For this review, take the finished solid that the model builds, in its own axes (mm). Coordinates: 2 decimals unless noted, no trailing zeros. Write each loop counter-clockwise with the first axis right and the second up, starting at its lowest first coordinate (ties: lowest second). Pieces come first, ordered by that corner, then holes. Notation, with made-up numbers: (72.25, -23.75) - (119.25, -23.75) arc R32 cw to (119.25, 3.25) - close; hole circle Ø10 at (29, 7). An arc over 180 degrees is marked (long way). Write each question's results on one line, items separated by ' | '.
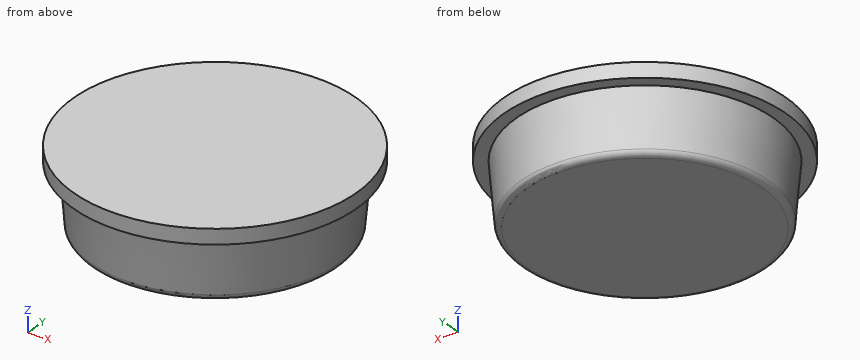
from build123d import *

# Parameters (mm, degrees)
SKETCH2_R           = 6.0325
BOSS_EXTRUDE1_DEPTH = 0.635
SKETCH1_R           = 5.2578
SKETCH3_R           = 5.4864
FILLET1_R           = 0.254


with BuildPart() as part:
    # Sketch2 → Boss-Extrude1 (new body)
    with BuildSketch(Plane.XY.offset(3.302)):
        Circle(SKETCH2_R)
    extrude(amount=-BOSS_EXTRUDE1_DEPTH)

    # Sketch1 → Loft1 section 0
    with BuildSketch(Plane.XY):
        Circle(SKETCH1_R)
    # Sketch3 → Loft1 section 1
    with BuildSketch(Plane(origin=(0, 0, 2.667), x_dir=(-1, 0, 0), z_dir=(0, 0, -1))):
        Circle(SKETCH3_R)
    loft()

    # Fillet1
    fillet1_edges = [part.edges().sort_by_distance(p)[0] for p in [
        (-5.2578, 0, 0),
    ]]
    fillet(fillet1_edges, radius=FILLET1_R)


solid = part.part
Q1. Wall thickness on line 1 along Z through (x, y) = (5.75, 0.5); line 2 along X through (y, z) = (1.75, 1.8); line 3 along X through (y, z) = (3.5, 0.55): over which ranges is each line inside the solid? List them lowest first. Write a range as from..to.
Results found:
line 1: 2.67..3.3 | line 2: -5.12..5.12 | line 3: -3.99..3.99
Q2. Take a section at A-A on x = 0. State the section outline as (y, z) points, plus the area to 3 significant figures.
Results found:
outline: (-6.03, 2.67) - (-5.49, 2.67) - (-5.28, 0.23) arc R0.25 ccw to (-5.02, 0) - (5.02, 0) arc R0.25 ccw to (5.28, 0.23) - (5.49, 2.67) - (6.03, 2.67) - (6.03, 3.3) - (-6.03, 3.3) - close | area: 36.3 mm2
Q3. Take a section at B-B on z = 3. State the section outline as (x, y) points (1 decimal).
Results found:
outline: circle Ø12.1 at (0, 0)
Q4. Take a section at C-C on z = 0.9. State the section outline as (x, y) points.
Results found:
outline: circle Ø10.67 at (0, 0)
Q5. For pin 1 (1 mm diameter, centred on x = -2, z = 2, fed in from -Y); pin 2 (1.5 mm diameter, centred on y = 0.5, z = 2, fed in from +X); pin 3 (1.5 mm diameter, centred on x = -4, z = 2.5, fed in from +Y); pin 4 (6 mm diameter, centred on x = -0.5, y = 0, fed in from -Z), all flat-tipped, find the tip position at first contact; note any pin that passes through.
Results found:
pin 1: y = -5.22 | pin 2: x = 6.03 | pin 3: y = 5.07 | pin 4: z = 0
